```python
from build123d import *

# Parameters (mm, degrees)
OUTER_START                           = -1.143
OUTER_CLAMP_LATCH_FILLET1_DEPTH       = 6.223
OUTER_START_2                         = 3.556
OUTER_CLAMP_LATCH_FILLET1_2_OUTLINE_R = 0.79375
OUTER_CLAMP_LATCH_FILLET1_2_DEPTH     = 1.524
OUTER_START_3                         = -0.508
OUTER_CLAMP_LATCH_FILLET1_3_OUTLINE_R = 0.79375
OUTER_CLAMP_LATCH_FILLET1_3_DEPTH     = 1.651
OUTER_CLAMP_LATCH_FILLET1_4_DEPTH     = 1.524
OUTER_START_4                         = 3.429
OUTER_CLAMP_LATCH_FILLET1_5_OUTLINE_R = 0.79375
OUTER_CLAMP_LATCH_FILLET1_5_DEPTH     = 0.127
OUTER_START_5                         = -7.112
OUTER_CLAMP_LATCH_FILLET1_6_DEPTH     = 1.5875
OUTER_START_6                         = -5.207
OUTER_CLAMP_LATCH_FILLET1_7_OUTLINE_R = 0.508
OUTER_CLAMP_LATCH_FILLET1_7_DEPTH     = 2.54
SKETCH1_W                             = 0.762
SKETCH1_H                             = 1.651
CUT_EXTRUDE1_DEPTH                    = 13.139632435
EXTRUDE1_START                        = -2.8575
SKETCH2_R                             = 0.508
EXTRUDE1_DEPTH                        = 2.8575
SKETCH2_3_R                           = 0.508
CUT_EXTRUDE2_DEPTH                    = 1.905


with BuildPart() as part:
    # <Outer Clamp Latch>-<Fillet1>: read off the stored shape, not the designer's step
    # <Outer Clamp Latch>-<Fillet1> outline → <Outer Clamp Latch>-<Fillet1> (new body)
    with BuildSketch(Plane.XY.offset(OUTER_START)):
        with BuildLine():
            Line((-4.445, -5.5245), (-4.445, -7.105634045))
            ThreePointArc((-4.445, -7.105634045), (-3.630142792, -6.693941899), (-3.302, -5.842))
            Line((-3.302, -5.842), (-3.302, -4.318))
            Line((-3.302, -4.318), (-4.064, -4.318))
            Line((-4.064, -4.318), (-4.064, -2.667))
            Line((-4.064, -2.667), (-7.62, -2.667))
            Line((-7.62, -2.667), (-7.62, -5.5245))
            Line((-7.62, -5.5245), (-4.445, -5.5245))
        make_face()
    extrude(amount=OUTER_CLAMP_LATCH_FILLET1_DEPTH)

    # Outer Clamp Latch_-_Fillet1 2 outline → Outer Clamp Latch_-_Fillet1 2 (add)
    # profile 1 of 2: a face of its own
    with BuildSketch(Plane.XY.offset(OUTER_START_2)):
        with BuildLine():
            Line((-7.62, -7.112), (-4.572, -7.112))
            ThreePointArc((-4.572, -7.112), (-4.508420276, -7.110407513), (-4.445, -7.105634045))
            Line((-4.445, -7.105634045), (-4.445, -5.5245))
            Line((-4.445, -5.5245), (-7.62, -5.5245))
            Line((-7.62, -5.5245), (-7.62, -7.112))
        make_face()
    # profile 2 of 2: a face of its own
    with BuildSketch(Plane.XY.offset(OUTER_START_2)):
        with BuildLine():
            Line((-7.62, -2.58093597), (-7.62, -2.667))
            Line((-7.62, -2.667), (-4.064, -2.667))
            Line((-4.064, -2.667), (-4.064, -2.6035))
            Line((-4.064, -2.6035), (-3.81, -2.6035))
            ThreePointArc((-3.81, -2.6035), (-2.343341242, -0.408490051), (-4.932532015, 0.106532015))
            Line((-4.932532015, 0.106532015), (-7.62, -2.58093597))
        make_face()
        with Locations((-3.81, -1.016)):
            Circle(OUTER_CLAMP_LATCH_FILLET1_2_OUTLINE_R, mode=Mode.SUBTRACT)
    extrude(amount=OUTER_CLAMP_LATCH_FILLET1_2_DEPTH)

    # Outer Clamp Latch_-_Fillet1 3 outline → Outer Clamp Latch_-_Fillet1 3 (add)
    with BuildSketch(Plane.XY.offset(OUTER_START_3)):
        with BuildLine():
            Line((-7.62, -2.58093597), (-7.62, -2.667))
            Line((-7.62, -2.667), (-4.064, -2.667))
            Line((-4.064, -2.667), (-4.064, -2.6035))
            Line((-4.064, -2.6035), (-3.81, -2.6035))
            ThreePointArc((-3.81, -2.6035), (-2.343341242, -0.408490051), (-4.932532015, 0.106532015))
            Line((-4.932532015, 0.106532015), (-7.62, -2.58093597))
        make_face()
        with Locations((-3.81, -1.016)):
            Circle(OUTER_CLAMP_LATCH_FILLET1_3_OUTLINE_R, mode=Mode.SUBTRACT)
    extrude(amount=OUTER_CLAMP_LATCH_FILLET1_3_DEPTH)

    # Outer Clamp Latch_-_Fillet1 4 outline → Outer Clamp Latch_-_Fillet1 4 (add)
    with BuildSketch(Plane.XY.offset(OUTER_START)):
        with BuildLine():
            Line((-7.62, -7.112), (-4.572, -7.112))
            ThreePointArc((-4.572, -7.112), (-4.508420276, -7.110407513), (-4.445, -7.105634045))
            Line((-4.445, -7.105634045), (-4.445, -5.5245))
            Line((-4.445, -5.5245), (-7.62, -5.5245))
            Line((-7.62, -5.5245), (-7.62, -7.112))
        make_face()
    extrude(amount=OUTER_CLAMP_LATCH_FILLET1_4_DEPTH)

    # Outer Clamp Latch_-_Fillet1 5 outline → Outer Clamp Latch_-_Fillet1 5 (add)
    with BuildSketch(Plane.XY.offset(OUTER_START_4)):
        with BuildLine():
            Line((-7.62, -2.58093597), (-7.62, -2.667))
            Line((-7.62, -2.667), (-4.064, -2.667))
            Line((-4.064, -2.667), (-4.064, -2.6035))
            Line((-4.064, -2.6035), (-3.81, -2.6035))
            ThreePointArc((-3.81, -2.6035), (-2.343341242, -0.408490051), (-4.932532015, 0.106532015))
            Line((-4.932532015, 0.106532015), (-7.62, -2.58093597))
        make_face()
        with Locations((-3.81, -1.016)):
            Circle(OUTER_CLAMP_LATCH_FILLET1_5_OUTLINE_R, mode=Mode.SUBTRACT)
    extrude(amount=OUTER_CLAMP_LATCH_FILLET1_5_DEPTH)

    # Outer Clamp Latch_-_Fillet1 6 outline → Outer Clamp Latch_-_Fillet1 6 (cut)
    with BuildSketch(Plane(origin=(0, 0, 0), x_dir=(1, 0, 0), z_dir=(0, 1, 0)).offset(OUTER_START_5)):
        with BuildLine():
            ThreePointArc((-4.445, -0.381), (-5.23875, 0.41275), (-6.0325, -0.381))
            Line((-6.0325, -0.381), (-4.445, -0.381))
        make_face()
        with BuildLine():
            ThreePointArc((-6.0325, -3.556), (-5.23875, -4.34975), (-4.445, -3.556))
            Line((-4.445, -3.556), (-6.0325, -3.556))
        make_face()
    extrude(amount=OUTER_CLAMP_LATCH_FILLET1_6_DEPTH, mode=Mode.SUBTRACT)

    # Outer Clamp Latch_-_Fillet1 7 outline → Outer Clamp Latch_-_Fillet1 7 (cut)
    with BuildSketch(Plane(origin=(0, 0, 0), x_dir=(1, 0, 0), z_dir=(0, 1, 0)).offset(OUTER_START_6)):
        with Locations((-5.715, -1.778)):
            Circle(OUTER_CLAMP_LATCH_FILLET1_7_OUTLINE_R)
    extrude(amount=OUTER_CLAMP_LATCH_FILLET1_7_DEPTH, mode=Mode.SUBTRACT)

    # Sketch1 → Cut-Extrude1 (cut, through all)
    with BuildSketch(Plane.XY.offset(5.08)):
        with Locations((-3.683, -5.1435)):
            Rectangle(SKETCH1_W, SKETCH1_H)
    extrude(amount=-CUT_EXTRUDE1_DEPTH, mode=Mode.SUBTRACT)

    # Sketch2 → Extrude1 (add)
    with BuildSketch(Plane(origin=(0, -2.667, 0), x_dir=(-1, 0, 0), z_dir=(0, 1, 0)).offset(EXTRUDE1_START)):
        with Locations((5.715, 2.794)):
            Circle(SKETCH2_R)
        with Locations((5.715, 1.778)):
            Circle(SKETCH2_R)
    extrude(amount=EXTRUDE1_DEPTH)

    # Sketch2<3> → Cut-Extrude2 (cut)
    with BuildSketch(Plane(origin=(0, -2.667, 0), x_dir=(-1, 0, 0), z_dir=(0, 1, 0))):
        with Locations(Location((5.715, 2.794, 0), (0, 0, 180))):
            Circle(SKETCH2_3_R)
    extrude(amount=-CUT_EXTRUDE2_DEPTH, mode=Mode.SUBTRACT)


solid = part.part
```
Check sheet for the modelled part. Datum: model origin and axes. Units: mm. A direction names the side the tool comes from. Give positions to 0.01 mm unless a question says otherwise; leave off trailing zeros. Order: outer loops, then holes, each group sorted by start corner. A loop starts at its lowest first (then second) coordinate and runs counter-clockwise, first axis right, second up. Notation, with made-up numbers: M 72.5,-27 L 125.5,-27 A20 cw 125.5,10 Z; hole C 33.5,37 d2. An arc over 180 degrees is marked long. Answer in a Markdown table with one row per item.
1) Access from +Z, -Z, +X, -X, +Y, -Y to the whole of each face (thin tool, end or side, straight path). Record for faces 5 (the flat face through (-4.064, -4, 2)), 6 (the flat face through (-4.445, -6, 2)), 7 (the flat face through (-6, -5.524, 2)), 8 (the flat face through (-5, -1, 1.143)), 9 (the flat face through (-5, -1, -0.508)).
Filled sheet:
| item | result |
|---|---|
| face 5 | +Z, -Z, +X |
| face 6 | -X, -Y |
| face 7 | -Y |
| face 8 | +X, -X, +Y |
| face 9 | -Z, +X, -X, +Y |
2) Gauge pin test, flat ends, axial feed: P1, Ø0.8, axis at x = -6, z = 2.5, coming from the +Y side; P2, Ø1, axis at x = -4, y = -1, coming from the -Z side; P3, Ø1.3, axis at x = -5.715, z = 2.794, coming from the -Y side; P4, Ø1.6, axis at x = -5.5, y = -0.5, coming from the -Z side. Record the tip position at first contact, or that the pin passes through.
Filled sheet:
| item | result |
|---|---|
| P1 | stops at y = -2.67 |
| P2 | passes through |
| P3 | stops at y = -5.52 |
| P4 | stops at z = -0.51 |
3) Cross-section at A-A, the plane y = -2. Enter the section's corners in (x, z), plus the area to 3 significant figures.
Filled sheet:
| item | result |
|---|---|
| outline | M -7.04,-0.51 L -2.56,-0.51 L -2.56,1.14 L -7.04,1.14 Z; M -7.04,3.43 L -2.56,3.43 L -2.56,5.08 L -7.04,5.08 Z |
| area | 14.8 mm2 |
4) Cross-section at B-B, the plane x = -2.6. Enter the section's corners in (y, z), plus the area to 3 significant figures.
Filled sheet:
| item | result |
|---|---|
| outline | M -2.04,-0.51 L 0.01,-0.51 L 0.01,1.14 L -2.04,1.14 Z; M -2.04,3.43 L 0.01,3.43 L 0.01,5.08 L -2.04,5.08 Z |
| area | 6.79 mm2 |
5) Release check for a two-part mould opening along X. For faces 1 (the flat face through (-6, -3, 5.08)), 2 (the flat face through (-6.26, -1.22, 4.24)), 3 (the cylindrical face through (-5.26, -6.33, 4.35)), 4 (the cylindrical face through (-3.91, -0.23, 0.31)) record: +X half, -X half, draft (parallel to the pull), parting line (faces both ways), or undercut.
Filled sheet:
| item | result |
|---|---|
| face 1 | draft |
| face 2 | -X half |
| face 3 | undercut |
| face 4 | undercut |
6) Thickness scan on L1, parallel to Z at x = -5.3, y = -2.5; L2, parallel to Y at x = -3.8, z = 0; L3, parallel to Z at x = -5.2, y = -6.5. Record the ranges inside material, lowest first. Write a range as [from, to].
Filled sheet:
| item | result |
|---|---|
| L1 | z = [-0.51, 1.14], [3.43, 5.08] |
| L2 | y = [-6.85, -5.97], [-2.6, -1.81], [-0.22, 0.57] |
| L3 | z = [-1.14, -0.41], [4.35, 5.08] |
7) Cross-section at C-C, the plane y = -5.75. Enter the section's corners in (x, z) (1 decimal), plus the area to 3 significant figures.
Filled sheet:
| item | result |
|---|---|
| outline | M -7.6,-1.1 L -4.1,-1.1 L -4.1,5.1 L -7.6,5.1 L -7.6,3.6 L -6,3.6 A0.8 cw -4.4,3.6 L -4.4,0.4 A0.8 cw -6,0.4 L -7.6,0.4 Z |
| area | 10.1 mm2 |
8) Cross-section at D-D, the plane x = -6.4. Enter the section's corners in (y, z), plus the area to 3 significant figures.
Filled sheet:
| item | result |
|---|---|
| outline | M -7.11,-1.14 L -2.67,-1.14 L -2.67,-0.51 L -1.36,-0.51 L -1.36,1.14 L -2.67,1.14 L -2.67,3.43 L -1.36,3.43 L -1.36,5.08 L -7.11,5.08 L -7.11,3.56 L -5.52,3.56 L -5.52,0.38 L -7.11,0.38 Z |
| area | 26.9 mm2 |
